Answer from the drawing. Dimensions are ordinates in mm from the lowest x, y and z of the part. A direction names the side the tool comes from. Give positions to 0.01 mm unless a question says otherwise; leave off trailing zeros. Loops run counter-clockwise (first coordinate to the right, second up) from the corner with the lowest first, then second, coordinate; pieces in that order, holes last. Notation, with made-up numbers: (31.5, 87) -> (82.5, 87) arc R29 cw to (82.5, 123) -> close; hole circle Ø11 at (2.5, 75). An arc over 180 degrees is marked (long way). Answer as CSV lines item,"result". Start each with the question number.
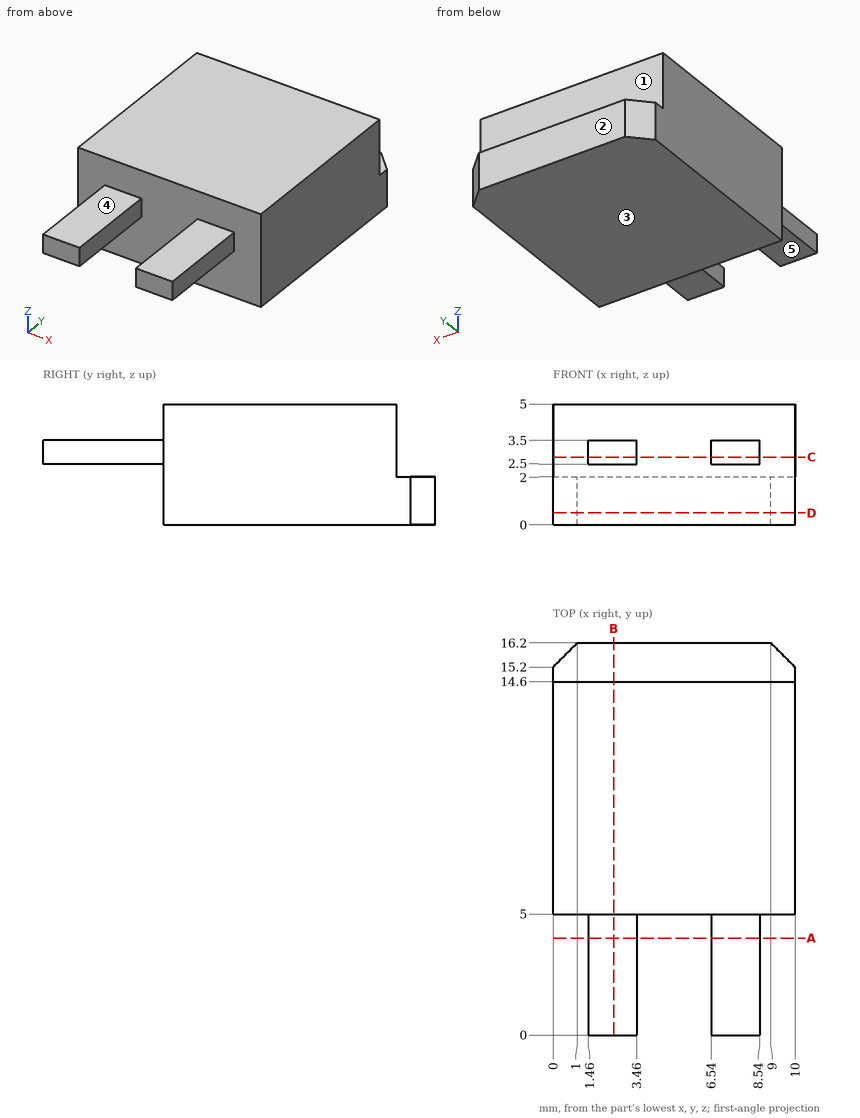
(1) Each of these flat-tipped pins is pushed along its axis until it touches: P1, Ø2, axis at x = 2.5, y = 3.5, coming from the -Z side; P2, Ø2.5, axis at x = 6, z = 3.5, coming from the +Y side; P3, Ø0.5, axis at y = 2, z = 3, coming from the +X side. Where does it stop, or does it pass through?
(2) Find section A-A on y = 4. Write down the section's boundary in (x, z), then the cut area to 3 significant figures.
(3) A tool of negligible diameter and unlimited length cuts with its end or side. For the marked faces 1, 2, 3, 4 and 5, from which of +Z, -Z, +X, -X, +Y, -Y can it reach the whole face along a straight path? Write none if from no direction.
(4) Find section D-D on z = 0.5. Write down the section's boundary in (x, y).
(5) Find section C-C on z = 2.8. Write down the section's boundary in (x, y).
(6) Find the intervals of material crossed by line 1 along Y through (x, z) = (3, 3.25); line 2 along Y through (x, z) = (2, 3.7); line 3 along Z through (x, y) = (1.5, 2.25), in increasing order. Write a range as from..to.
(7) Find section B-B on x = 2.5. Write down the section's boundary in (y, z), then the cut area to 3 significant figures.
Answer block:
1,P1,"stops at z = 2.5"
1,P2,"stops at y = 14.6"
1,P3,"stops at x = 8.54"
2,outline,"(1.46, 2.5) -> (3.46, 2.5) -> (3.46, 3.5) -> (1.46, 3.5) -> close; (6.54, 2.5) -> (8.54, 2.5) -> (8.54, 3.5) -> (6.54, 3.5) -> close"
2,area,"4.00 mm2"
3,face 1,"+Z, +X, -X, +Y"
3,face 2,"+Z, -Z, +X, -X, +Y"
3,face 3,"-Z, +X, -X, +Y, -Y"
3,face 4,"+Z, +X, -X, -Y"
3,face 5,"-Z, +X, -X, -Y"
4,outline,"(0, 5) -> (10, 5) -> (10, 15.2) -> (9, 16.2) -> (1, 16.2) -> (0, 15.2) -> close"
5,outline,"(0, 5) -> (1.46, 5) -> (1.46, 0) -> (3.46, 0) -> (3.46, 5) -> (6.54, 5) -> (6.54, 0) -> (8.54, 0) -> (8.54, 5) -> (10, 5) -> (10, 14.6) -> (0, 14.6) -> close"
6,line 1,"y = 0..14.6"
6,line 2,"y = 5..14.6"
6,line 3,"z = 2.5..3.5"
7,outline,"(0, 2.5) -> (5, 2.5) -> (5, 0) -> (16.2, 0) -> (16.2, 2) -> (14.6, 2) -> (14.6, 5) -> (5, 5) -> (5, 3.5) -> (0, 3.5) -> close"
7,area,"56.2 mm2"
